```python
from build123d import *

# Parameters (mm, degrees)
F0_W      = 152.4
F0_H      = 44.45
F1_DEPTH  = 38.1
F3_DEPTH  = 87.376
F4_W      = 34.063664
F4_H      = 24.459008
F5_DEPTH  = 8.636
F6_W      = 1.7526
F6_H      = 12.453256
F7_DEPTH  = 71.12
F8_W      = 1.7526
F8_H      = 5.531359
F9_DEPTH  = 63.2968
F10_R     = 1.848563
F10_R_2   = 0.78284
F11_DEPTH = 2.8194
F12_R     = 1.867057
F12_R_2   = 0.756279
F13_DEPTH = 3.2766
F14_W     = 2.55886
F14_H     = 11.105731
F15_DEPTH = 2.286


with BuildPart() as f1:
    # F0 (on Top) → F1 (new body)
    with BuildSketch(Plane.XY):
        Rectangle(F0_W, F0_H)
    extrude(amount=F1_DEPTH)

    # F2 (on face) → F3 (cut)
    with BuildSketch(Plane.XZ.offset(22.225)):
        Polygon((-92.090726, 33.964641), (-76.2, 0), (-47.134604, 17.130854), (33.073444, 17.130854), (61.393816, 22.676103), (76.2, 32.57833), (86.743511, 41.292287), (-31.291042, 57.729989), align=None)
    extrude(amount=-F3_DEPTH, mode=Mode.SUBTRACT)

    # F4 (on face) → F5 (cut)
    with BuildSketch(Plane.XY.offset(17.130854)):
        Rectangle(F4_W, F4_H)
    extrude(amount=-F5_DEPTH, mode=Mode.SUBTRACT)

    # F6 (on face) → F7 (cut)
    with BuildSketch(Plane.XZ.offset(22.225)):
        with Locations((-55.441208, -2.873828)):
            Rectangle(F6_W, F6_H)
    extrude(amount=-F7_DEPTH, mode=Mode.SUBTRACT)

    # F8 (on face) → F9 (cut)
    with BuildSketch(Plane.XZ.offset(22.225)):
        with Locations((58.901841, 0.58712)):
            Rectangle(F8_W, F8_H)
    extrude(amount=-F9_DEPTH, mode=Mode.SUBTRACT)

    # F10 (on face) → F11 (join)
    with BuildSketch(Plane.YZ.offset(76.2)):
        with Locations((-15.979337, 4.065371)):
            Circle(F10_R)
        with Locations((-15.979337, 4.065371)):
            Circle(F10_R_2, mode=Mode.SUBTRACT)
    extrude(amount=F11_DEPTH)

    # F12 (on face) → F13 (join)
    with BuildSketch(Plane.YZ.offset(76.2)):
        with Locations((14.432833, 3.567662)):
            Circle(F12_R)
        with Locations((14.432833, 3.567662)):
            Circle(F12_R_2, mode=Mode.SUBTRACT)
    extrude(amount=F13_DEPTH)

    # F14 (on face) → F15 (join)
    with BuildSketch(Plane.YZ.offset(76.2)):
        Polygon((-5.871529, 25.838383), (-2.55886, 25.838383), (0, 25.838383), (3.520685, 25.838383), (3.520685, 28.528722), (-5.871529, 28.528722), align=None)
        with Locations((-1.27943, 20.285518)):
            Rectangle(F14_W, F14_H)
    extrude(amount=F15_DEPTH)


solid = f1.part
```
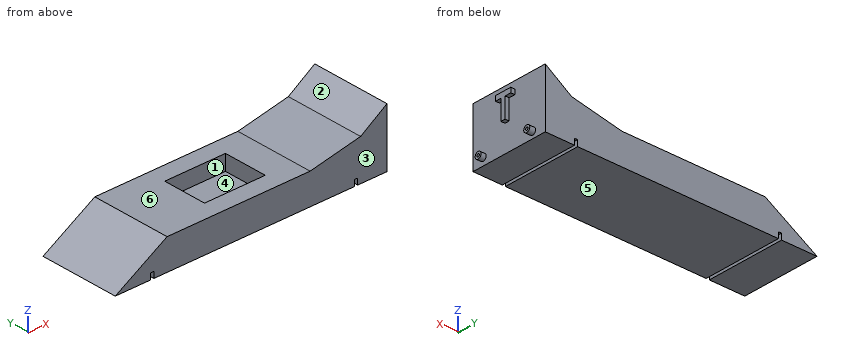
Work out the finished part from the listing and answer in its coordinate system (mm). Face numbers are marked on the shaded views. A direction names the side the tool comes from. Round coordinates to 2 decimals unless told otherwise and drop trailing zeros. Write each loop counter-clockwise with the first axis right and the second up, starting at its lowest first coordinate (ties: lowest second). Pieces come first, ordered by that corner, then holes.
1) Which of the six approach directions +Z, -Z, +X, -X, +Y, -Y give full straight-line access (tool end or side, diameter ignored) to the marked faces 5 and 6?
2) A cutting plane is placed at A-A on x = 7. Determine the outline of the cut face in (y, z) (1 decimal), and give its area (3 significant figures).
3) A cutting plane is placed at C-C on z = 19.5. Determine the outline of the cut face in (x, y) (3 decimals), and give its area (4 significant figures).
4) Flat-ended cylindrical pins translate along their axes: P1, Ø4, axis at x = 36, y = 3, coming from the +Z side; P2, Ø1.1, axis at x = 77.5, z = 18.5, coming from the +Y side; P3, Ø3, axis at y = 7, z = 11.5, coming from the -X side; P4, Ø10, axis at x = -33, z = 19.5, coming from the +Y side (3 decimals). Find the tip coordinate at first contact, or state that the pin passes through.
5) A cutting plane is placed at B-B on y = 9. Determine the outline of the cut face in (x, z).
6) Consider probe 1 along Z at (x, y) = (-16, -11); probe 2 along Z at (x, y) = (25, 19.5); probe 3 along X at (y, z) = (7, 13.5). Determine where each line is inside the solid, lowest interval first.
7) A cutting plane is placed at D-D on x = -35.5. Determine the outline of the cut face in (y, z) (3 decimals).
8) Determine the mould class of the marked faces 1, 2, 3 and 4 for opening direction Y: pulls with the +Y half, pulls with the -Y half, needs draft (parallel to the pull), parting line crosses it, or undercut.
Entries:
1. face 5: -Z, +X, -X, +Y, -Y
1. face 6: +Z, -X, +Y, -Y
2. outline: (-22.2, 0) - (22.2, 0) - (22.2, 17.1) - (12.2, 17.1) - (12.2, 8.5) - (-12.2, 8.5) - (-12.2, 17.1) - (-22.2, 17.1) - close
2. area: 550 mm2
3. outline: (45.173, -22.225) - (76.2, -22.225) - (76.2, -2.559) - (78.486, -2.559) - (78.486, 0) - (76.2, 0) - (76.2, 22.225) - (45.173, 22.225) - close
3. area: 1,385 mm2
4. P1: stops at z = 18.1
4. P2: stops at y = 0
4. P3: stops at x = -59.23
4. P4: stops at y = 22.225
5. outline: (-76.2, 0) - (-56.32, 0) - (-56.32, 3.35) - (-54.56, 3.35) - (-54.56, 0) - (58.03, 0) - (58.03, 3.35) - (59.78, 3.35) - (59.78, 0) - (76.2, 0) - (76.2, 32.58) - (61.39, 22.68) - (33.07, 17.13) - (17.03, 17.13) - (17.03, 8.49) - (-17.03, 8.49) - (-17.03, 17.13) - (-47.13, 17.13) - close
6. probe 1: z = 0 to 8.49
6. probe 2: z = 0 to 17.13
6. probe 3: x = -53.29 to -17.03, 17.03 to 76.2
7. outline: (-22.225, 0) - (22.225, 0) - (22.225, 17.131) - (-22.225, 17.131) - close
8. face 1: undercut
8. face 2: needs draft
8. face 3: pulls with the -Y half
8. face 4: undercut
